Part model, mm, in its own coordinate system. Face numbers are marked on the shaded views. A direction names the side the tool comes from. Coordinates: 2 decimals unless noted, no trailing zeros. Write each loop counter-clockwise with the first axis right and the second up, starting at its lowest first coordinate (ties: lowest second). Pieces come first, ordered by that corner, then holes. Notation, with made-up numbers: M -16.5,16 L 33.5,16 A17 cw 33.5,39 Z; hole C 28.5,64.5 d6. An arc over 180 degrees is marked long. Use a Markdown table: item, result. Add a question column.
Q1. Slice it at D-D on y = 11.15. Write the cut outline in (x, z), then the cut area to 3 significant figures.
Q2. Mould opens along X. For the marked faces 1, 2 and 3 say: released by +X, released by -X, zero draft, split by the parting line, or undercut.
Q3. Slice it at B-B on z = 1. Write the cut outline in (x, y).
Q4. Wall check: L1, parallel to Z at x = 21.75, y = 9; L2, parallel to Z at x = 22.5, y = 10.5; L3, parallel to X at y = 11.15, z = 1.9. Give the ranges that are in metal, low to high. Write a range as from..to.
Q5. Slice it at C-C on y = 7. Write the cut outline in (x, z), then the cut area to 3 significant figures.
Q6. Slice it at A-A on x = 13.75. Write the cut outline in (y, z), then the cut area to 3 significant figures.
Q7. Pin check, flat tips, straight feed: pin 1 Ø2 at (y, z) = (11.15, 9) entering from -X; pin 2 Ø10 at (y, z) = (10.5, 10) entering from +X; pin 3 Ø2 at (y, z) = (32.375, 9) entering from +X. Stop position of each tip, or through.
Q8. Tool access for the marked faces 4 and 5: list every direction of +Z, -Z, +X, -X, +Y, -Y with a clear straight run to the whole face (end or side of a thin tool).
from build123d import *

# Parameters (mm, degrees)
BOSS_EXTRUDE1_DEPTH = 35
SKETCH2_R           = 1.75
SKETCH2_W           = 11.6
SKETCH2_H           = 22.75
CUT_EXTRUDE1_DEPTH  = 4
SKETCH3_R           = 1.25
CUT_EXTRUDE2_DEPTH  = 32
SKETCH4_R           = 1
CUT_EXTRUDE3_DEPTH  = 4


with BuildPart() as part:
    # Sketch1 → Boss-Extrude1 (new body)
    with BuildSketch(Plane(origin=(0, 0, 0), x_dir=(1, 0, 0), z_dir=(0, 1, 0))):
        Polygon((15, 0), (15, -1.59), (1.59, -1.59), (1.59, -16.41), (22.41, -16.41), (22.41, -1.59), (19, -1.59), (19, 0), (24, 0), (24, -18), (0, -18), (0, 0), align=None)
    extrude(amount=BOSS_EXTRUDE1_DEPTH)

    # Sketch2 → Cut-Extrude1 (cut)
    with BuildSketch(Plane(origin=(24, 0, 0), x_dir=(0, 0, -1), z_dir=(1, 0, 0))):
        with Locations((-9, 32.375)):
            Circle(SKETCH2_R)
        with Locations((-9, 2.625)):
            Circle(SKETCH2_R)
        with Locations((-9, 17.5)):
            Rectangle(SKETCH2_W, SKETCH2_H)
    extrude(amount=-CUT_EXTRUDE1_DEPTH, mode=Mode.SUBTRACT)

    # Sketch3 → Cut-Extrude2 (cut)
    with BuildSketch(Plane.ZY):
        with Locations((9, 11.15)):
            Circle(SKETCH3_R)
    extrude(amount=-CUT_EXTRUDE2_DEPTH, mode=Mode.SUBTRACT)

    # Sketch4 → Cut-Extrude3 (cut)
    with BuildSketch(Plane(origin=(0, 0, 0), x_dir=(-1, 0, 0), z_dir=(0, 0, -1))):
        with Locations((-11.5, 11.15)):
            Circle(SKETCH4_R)
        with Locations((-21.5, 11.15)):
            Circle(SKETCH4_R)
    extrude(amount=-CUT_EXTRUDE3_DEPTH, mode=Mode.SUBTRACT)


solid = part.part
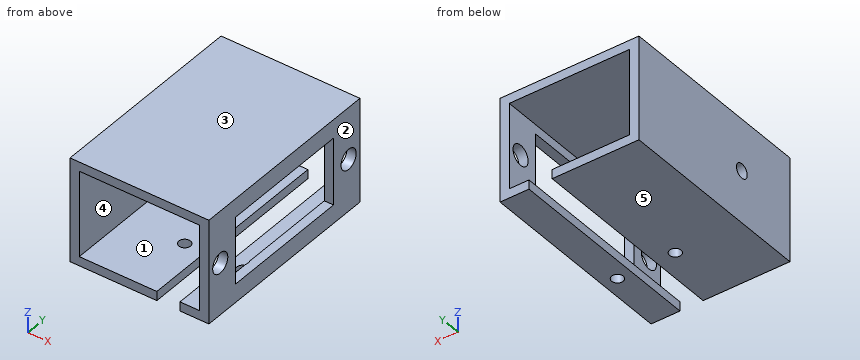
Recorded:
| question | item | result |
|---|---|---|
| 1 | outline | M 0,0 L 10.5,0 L 10.5,1.59 L 1.59,1.59 L 1.59,7.75 L 0,7.75 Z; M 0,10.25 L 1.59,10.25 L 1.59,16.41 L 22.41,16.41 L 22.41,14.8 L 24,14.8 L 24,18 L 0,18 Z; M 12.5,0 L 15,0 L 15,1.59 L 12.5,1.59 Z; M 19,0 L 20.5,0 L 20.5,1.59 L 19,1.59 Z; M 22.5,0 L 24,0 L 24,3.2 L 22.5,3.2 Z |
| 1 | area | 88.2 mm² |
| 2 | face 1 | undercut |
| 2 | face 2 | released by +X |
| 2 | face 3 | zero draft |
| 3 | outline | M 0,0 L 15,0 L 15,35 L 0,35 Z; M 19,0 L 24,0 L 24,35 L 19,35 Z; hole C 11.5,11.15 d2; hole C 21.5,11.15 d2 |
| 4 | L1 | 0..1.59, 16.41..18 |
| 4 | L2 | 0..3.2, 14.8..18 |
| 4 | L3 | 0..1.59, 22.5..24 |
| 5 | outline | M 0,0 L 15,0 L 15,1.59 L 1.59,1.59 L 1.59,16.41 L 22.41,16.41 L 22.41,14.8 L 24,14.8 L 24,18 L 0,18 Z; M 19,0 L 24,0 L 24,3.2 L 22.41,3.2 L 22.41,1.59 L 19,1.59 Z |
| 5 | area | 98.6 mm² |
| 6 | outline | M 0,0 L 35,0 L 35,1.59 L 0,1.59 Z; M 0,16.41 L 35,16.41 L 35,18 L 0,18 Z |
| 6 | area | 111 mm² |
| 7 | pin 1 | through |
| 7 | pin 2 | x = 24 |
| 7 | pin 3 | x = 1.59 |
| 8 | face 4 | +Y, -Y |
| 8 | face 5 | -Z, +X, -X, +Y, -Y |
